For this review, use the dimensioned drawing (mm, ordinates from the lowest corner) and the shaded views. Coordinates: 2 decimals unless noted, no trailing zeros. Order: outer loops, then holes, each group sorted by start corner. A loop starts at its lowest first (then second) coordinate and runs counter-clockwise, first axis right, second up. Notation, with made-up numbers: M 35,8.25 L 44,8.25 A15 cw 44,20.25 Z; hole C -5,22.25 d11. An arc over 180 degrees is marked long. Answer in a Markdown table with one row per item.
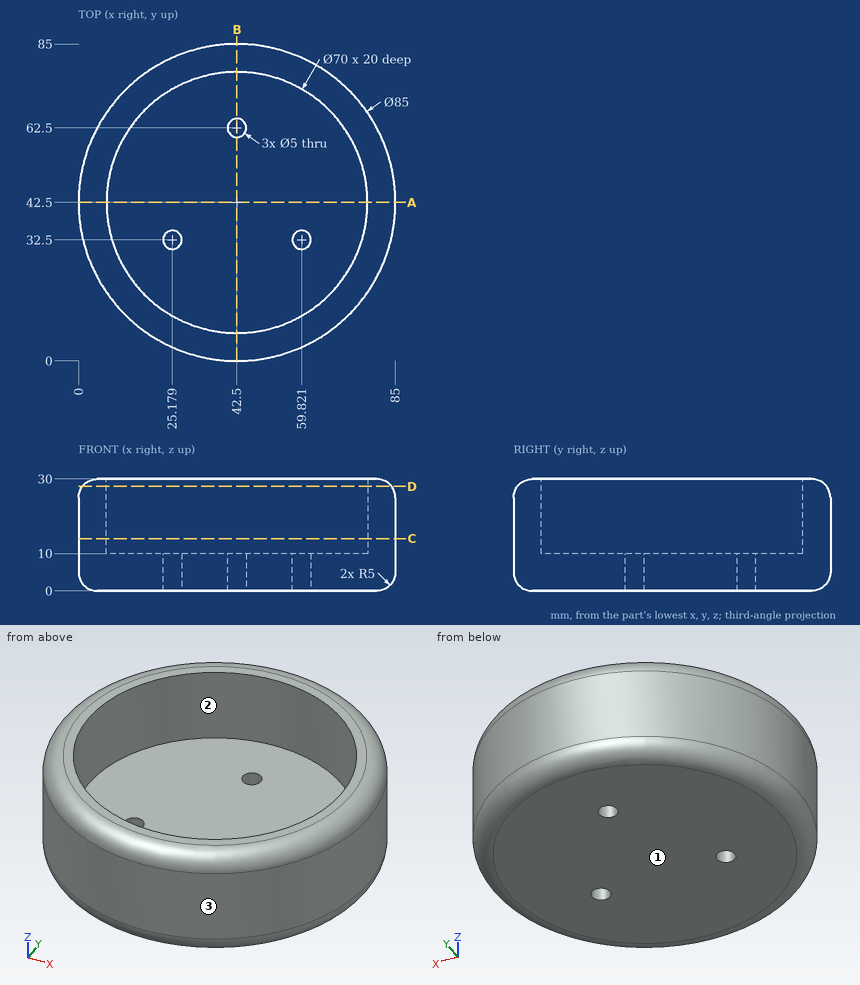
(1) Insertion check: pin 1 Ø5 at (y, z) = (57.5, 9) entering from +X; pin 2 Ø8 at (x, y) = (59.82, 32.5) entering from +Z; pin 3 Ø1 at (x, z) = (69.5, 22.5) entering from +Y (1 decimal). Each pin has a flat end and moves straight along its axis. Give the tip position at first contact, or say it passes through.
Return value:
| item | result |
|---|---|
| pin 1 | stops at x = 83.12 |
| pin 2 | stops at z = 10 |
| pin 3 | stops at y = 75.7 |
(2) Add section B-B, the plane x = 42.5. Give the boundary of the cut face in (y, z).
Return value:
| item | result |
|---|---|
| outline | M 0,5 A5 ccw 5,0 L 60,0 L 60,10 L 7.5,10 L 7.5,30 L 5,30 A5 ccw 0,25 Z; M 65,0 L 80,0 A5 ccw 85,5 L 85,25 A5 ccw 80,30 L 77.5,30 L 77.5,10 L 65,10 Z |
(3) Add section D-D, the plane z = 28. Give the boundary of the cut face in (x, y).
Return value:
| item | result |
|---|---|
| outline | C 42.5,42.5 d83; hole C 42.5,42.5 d70 |
(4) Add section A-A, the plane y = 42.5. Give the boundary of the cut face in (x, z).
Return value:
| item | result |
|---|---|
| outline | M 0,5 A5 ccw 5,0 L 80,0 A5 ccw 85,5 L 85,25 A5 ccw 80,30 L 77.5,30 L 77.5,10 L 7.5,10 L 7.5,30 L 5,30 A5 ccw 0,25 Z |
(5) Add section C-C, the plane z = 14. Give the boundary of the cut face in (x, y), and give its area (3 significant figures).
Return value:
| item | result |
|---|---|
| outline | C 42.5,42.5 d85; hole C 42.5,42.5 d70 |
| area | 1,830 mm2 |
(6) Draft analysis for pull direction X (two halves, no side actions). For the marked faces 1, 2 and 3, state which applies: pulls with the +X half, pulls with the -X half, needs draft (parallel to the pull), parting line crosses it, or undercut.
Return value:
| item | result |
|---|---|
| face 1 | needs draft |
| face 2 | undercut |
| face 3 | parting line crosses it |
(7) For line 1 along Z through (x, y) = (27, 71); line 2 along Y through (x, z) = (42.5, 7.25); line 3 along Y through (x, z) = (48, 20) (1 decimal), list the stretches that pass through material, from the lowest coordinate up. Write a range as from..to.
Return value:
| item | result |
|---|---|
| line 1 | z = 0..10 |
| line 2 | y = 0..60, 65..85 |
| line 3 | y = 0.4..7.9, 77.1..84.6 |
